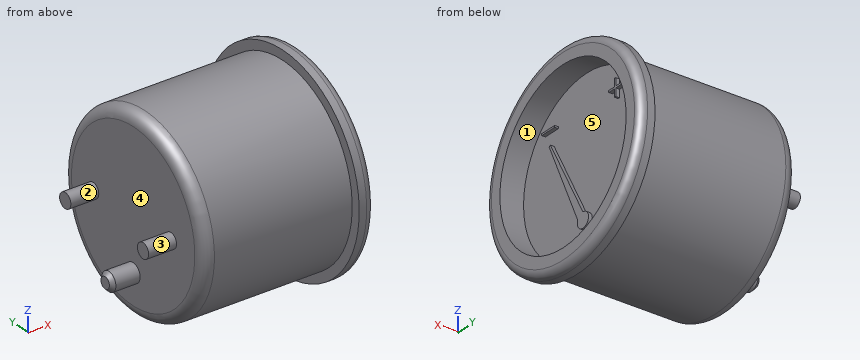
Solid Edge part; units mm, degrees
sketch "Sketch1" plane through (0, 0, 0) normal (1, 0, 0) x (0, 1, 0)
  circle A0 centre (-26.289, 4.8888) radius 25
extrude "Protrusion1" add sketch "Sketch1" against normal blind 40
sketch "Sketch2" plane through (0, -26.289, 4.8888) normal (1, 0, 0) x (0, 0, 1)
  circle A0 centre (0, 0) radius 27.5
extrude "ExtrudedProtrusion_2" add sketch "Sketch2" along normal blind 4
fillet "Round_1" radius 2 1 edges at (4, -26.289, -22.6112)
fillet "Round_2" radius 3 1 edges at (-40, -51.289, 4.8888)
sketch "Sketch3" plane through (-40, -26.289, 4.8888) normal (-1, 0, 0) x (0, -1, 0)
  circle A0 centre (-14.2428, 0) radius 2
  circle A1 centre (13.4912, 0) radius 2
  circle A2 centre (0, -13.867) radius 2.5
extrude "ExtrudedProtrusion_3" add sketch "Sketch3" along normal blind 7.5
chamfer "Chamfer_1" distance 1 angle 45 1 edges at (-47.5, -23.789, -8.9782)
sketch "Sketch4" plane through (4, -26.289, 4.8888) normal (1, 0, 0) x (0, 1, 0)
  circle A0 centre (0, 0) radius 22.5
extrude "ExtrudedCutout_1" cut sketch "Sketch4" against normal blind 6.35
sketch "Sketch5" plane through (-2.35, -26.289, 4.8888) normal (1, 0, 0) x (0, 1, 0)
  line L0 (0, -11.867) -> (-11.6013, 9.6746)
  line L1 (-12.0271, 9.3319) -> (-11.6013, 9.6746)
  line L2 (-12.0271, 9.3319) -> (-1.8479, -13.1021)
  arc A0 (-1.8479, -13.1021) -> (0, -11.867) centre (0, -13.867) ccw
  line L3 (-14.6973, 13.3557) -> (-10.0815, 13.3557)
  line L4 (-10.0815, 13.3557) -> (-10.0815, 13.8208)
  line L5 (-10.0815, 13.8208) -> (-14.6973, 13.8208)
  line L6 (-14.6973, 13.8208) -> (-14.6973, 13.3557)
  line L7 (11.7077, 13.3557) -> (13.7958, 13.3557)
  line L8 (13.7958, 13.3557) -> (13.7958, 13.8208)
  line L9 (13.7958, 13.8208) -> (11.7077, 13.8208)
  line L10 (11.7077, 13.8208) -> (11.7077, 15.8834)
  line L11 (11.7077, 15.8834) -> (11.2426, 15.8834)
  line L12 (11.2426, 15.8834) -> (11.2426, 13.8208)
  line L13 (11.2426, 13.8208) -> (9.18, 13.8208)
  line L14 (9.18, 13.8208) -> (9.18, 13.3557)
  line L15 (9.18, 13.3557) -> (11.2426, 13.3557)
  line L16 (11.2426, 13.3557) -> (11.2426, 11.2676)
  line L17 (11.2426, 11.2676) -> (11.7077, 11.2676)
  line L18 (11.7077, 11.2676) -> (11.7077, 13.3557)
  line L19 (9.18, 13.3557) -> (13.7958, 13.3557)
  line L20 (13.7958, 13.3557) -> (13.7958, 13.8208)
  line L21 (13.7958, 13.8208) -> (9.18, 13.8208)
  line L22 (9.18, 13.8208) -> (9.18, 13.3557)
  line L23 (11.7077, 11.2676) -> (11.7077, 15.8834)
  line L24 (11.7077, 15.8834) -> (11.2426, 15.8834)
  line L25 (11.2426, 15.8834) -> (11.2426, 11.2676)
  line L26 (11.2426, 11.2676) -> (11.7077, 11.2676)
extrude "ExtrudedProtrusion_4" add sketch "Sketch5" along normal blind 1
Verification items for the finished model (mm, model axes). Face numbers are marked on the shaded views. A direction names the side the tool comes from. Round coordinates to 2 decimals unless told otherwise and drop trailing zeros. Write each loop counter-clockwise with the first axis right and the second up, starting at its lowest first coordinate (ties: lowest second). Pieces come first, ordered by that corner, then holes. Notation, with made-up numbers: (-26, 88.5) -> (-13, 88.5) arc R18 cw to (-13, 113.5) -> close; hole circle Ø7 at (74, -26). An arc over 180 degrees is marked (long way). Write each question's results on one line, items separated by ' | '.
Q1. Thickness scan on probe 1 along Y at (x, z) = (-1.5, 17.5); probe 2 along Y at (x, z) = (1.5, -12); probe 3 along X at (y, z) = (-27, -4.5). Record the ranges inside material, lowest first.
Derived:
probe 1: y = -47.88 to -44.92, -15.05 to -14.58, -7.66 to -4.7 | probe 2: y = -47.99 to -41.16, -11.42 to -4.59 | probe 3: x = -40 to -2.35
Q2. Go/stop test with flat-tipped pins: pin 1 Ø3 at (y, z) = (-19.5, 21.5) entering from +X; pin 2 Ø0.5 at (x, y) = (-1.5, -14.5) entering from +Z; pin 3 Ø4 at (y, z) = (-5, -16.5) entering from +X; pin 4 Ø5 at (x, z) = (-10, -11) entering from +Y. Record where each tip stops, or that it passes through.
Derived:
pin 1: stops at x = -2.35 | pin 2: stops at z = 27.07 | pin 3: passes through | pin 4: stops at y = -5.18
Q3. Sectioned sample at A-A, the plane x = -7. Record the boundary of the cut face in (y, z), and give its area (3 significant figures).
Derived:
outline: circle Ø50 at (-26.29, 4.89) | area: 1,960 mm²
Q4. Access from +Z, -Z, +X, -X, +Y, -Y to the whole of each face (thin tool, end or side, straight path). Record for the marked faces 1 and 2.
Derived:
face 1: +X | face 2: -X
Q5. Draft check along Z on the marked faces 3, 4 and 5. Enter one of: released by +Z, released by -Z, zero draft, split by the parting line, or undercut.
Derived:
face 3: split by the parting line | face 4: zero draft | face 5: undercut
